Could you check a few things on this model? Use its own coordinates, in mm. Face numbers are marked on the shaded views. A direction names the side the tool comes from. Coordinates: 2 decimals unless noted, no trailing zeros. Loops run counter-clockwise (first coordinate to the right, second up) from the corner with the lowest first, then second, coordinate; pieces in that order, holes last. Notation, with made-up numbers: M 3.25,0.25 L 12.25,0.25 A21 cw 12.25,36.25 Z; hole C 82.25,47.5 d10. An arc over 180 degrees is marked long. Return JSON: item names as keys, results as strings. Group by question number.
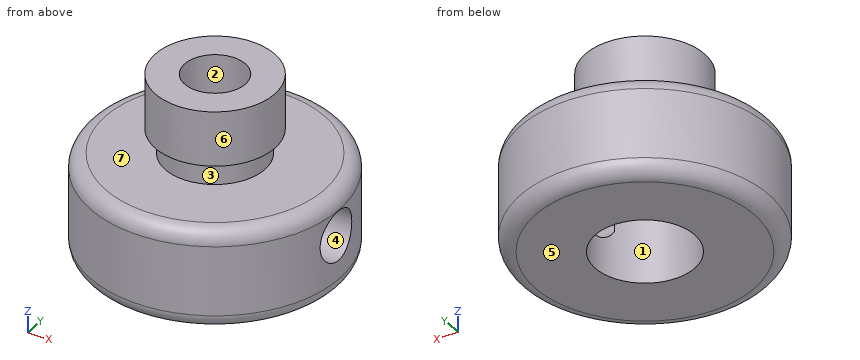
from build123d import *

# Parameters (mm, degrees)
ESQUISSE1_R             = 12.5
BASE_EXTRUSION_DEPTH    = 10
ESQUISSE2_R             = 6
BOSS_EXTRU_1_DEPTH      = 8
ESQUISSE3_R             = 3.05
ENL_V_MAT_EXTRU_1_DEPTH = 26.228951623
ESQUISSE4_R             = 5
ENL_V_MAT_EXTRU_2_DEPTH = 8
ESQUISSE5_W             = 2.5
ESQUISSE5_H             = 2
CONG_1_R                = 1.5
ESQUISSE7_R             = 2.5
ENL_V_MAT_EXTRU_4_DEPTH = 8


with BuildPart() as part:
    # Esquisse1 → Base-Extrusion (new body)
    with BuildSketch(Plane.XY):
        Circle(ESQUISSE1_R)
    extrude(amount=BASE_EXTRUSION_DEPTH)

    # Esquisse2 → Boss.-Extru.1 (add)
    with BuildSketch(Plane.XY.offset(10)):
        Circle(ESQUISSE2_R)
    extrude(amount=BOSS_EXTRU_1_DEPTH)

    # Esquisse3 → Enlèv. mat.-Extru.1 (cut, through all)
    with BuildSketch(Plane.XY.offset(18)):
        Circle(ESQUISSE3_R)
    extrude(amount=-ENL_V_MAT_EXTRU_1_DEPTH, mode=Mode.SUBTRACT)

    # Esquisse4 → Enlèv. mat.-Extru.2 (cut)
    with BuildSketch(Plane(origin=(0, 0, 0), x_dir=(-1, 0, 0), z_dir=(0, 0, -1))):
        Circle(ESQUISSE4_R)
    extrude(amount=-ENL_V_MAT_EXTRU_2_DEPTH, mode=Mode.SUBTRACT)

    # Esquisse5 → Enlever de la matière-Révolution1 (revolve, cut)
    with BuildSketch(Plane(origin=(0, 0, 0), x_dir=(0, 0, -1), z_dir=(1, 0, 0)), mode=Mode.PRIVATE) as enlever_de_la_mati_re_r_volution1_sk:
        with Locations((-11.25, 6)):
            Rectangle(ESQUISSE5_W, ESQUISSE5_H)
    revolve(enlever_de_la_mati_re_r_volution1_sk.sketch.rotate(Axis((0, 0, 21.399826727), (0, 0, -1)), 90), axis=Axis((0, 0, 21.399826727), (0, 0, -1)), mode=Mode.SUBTRACT)

    # Congé1
    cong_1_edges = [part.edges().sort_by_distance(p)[0] for p in [
        (-12.5, 0, 0),
        (-12.5, 0, 10),
    ]]
    fillet(cong_1_edges, radius=CONG_1_R)

    # Esquisse7 → Enlèv. mat.-Extru.4 (cut)
    with BuildSketch(Plane(origin=(12.5, 0, 0), x_dir=(0, 0, -1), z_dir=(1, 0, 0))):
        with Locations((-5.942386831, 0)):
            Circle(ESQUISSE7_R)
    extrude(amount=-ENL_V_MAT_EXTRU_4_DEPTH, mode=Mode.SUBTRACT)


solid = part.part
(1) For the marked faces 5, 6 and 7, which set-ups out of +Z, -Z, +X, -X, +Y, -Y let a thin tool reach every point of the face, with its end or its side?
(2) Imagine slicing it at A-A, the plane x = 0. Write out the boundary of the cut face in (y, z), then the cut area to 3 significant figures.
(3) Will these pins go through, and if not, where does the flat tip stop? P1, Ø1.5, axis at x = 3.5, z = 15, coming from the +Y side; P2, Ø2, axis at x = 3.5, z = 15, coming from the -Y side; P3, Ø1, axis at y = 2.5, z = 5, coming from the -X side; P4, Ø3.5, axis at x = 0, y = 0, coming from the -Z side.
(4) Imagine slicing it at B-B, the plane y = 0. Write out the boundary of the cut face in (x, z).
(5) Imagine slicing it at D-D, the plane z = 11.25. Write out the boundary of the cut face in (x, y).
(6) Imagine slicing it at C-C, the plane z = 14. Write out the boundary of the cut face in (x, y).
(7) We'd pull the mould along X, two halves only. Please class the marked faces 1, 2, 3 and 4: +X half, -X half, draft (parallel to the pull), parting line (faces both ways), or undercut.
(8) If I drill on L1, parallel to Z at x = -5, y = -0.75; L2, parallel to Z at x = 8, y = 0; L3, parallel to Y at x = 0, z = 12.25, over which ranges is the centre line in solid material (lowest first)? Write a range as [from, to].
Checks:
{
 "1": {"face 5": "-Z, +X, -X, +Y, -Y", "face 6": "+Z", "face 7": "none"},
 "2": {"outline": "M -12.5,1.5 A1.5 ccw -11,0 L -5,0 L -5,8 L -3.05,8 L -3.05,18 L -6,18 L -6,12.5 L -5,12.5 L -5,10 L -11,10 A1.5 ccw -12.5,8.5 Z; M 3.05,8 L 5,8 L 5,0 L 11,0 A1.5 ccw 12.5,1.5 L 12.5,8.5 A1.5 ccw 11,10 L 5,10 L 5,12.5 L 6,12.5 L 6,18 L 3.05,18 Z", "area": "198 mm²"},
 "3": {"P1": "y = 5.33", "P2": "y = -5.45", "P3": "x = -12.34", "P4": "through"},
 "4": {"outline": "M -12.5,1.5 A1.5 ccw -11,0 L -5,0 L -5,8 L -3.05,8 L -3.05,18 L -6,18 L -6,12.5 L -5,12.5 L -5,10 L -11,10 A1.5 ccw -12.5,8.5 Z; M 3.05,8 L 4.5,8 L 4.5,8.44 L 12.5,8.44 L 12.5,8.5 A1.5 ccw 11,10 L 5,10 L 5,12.5 L 6,12.5 L 6,18 L 3.05,18 Z; M 5,0 L 11,0 A1.5 ccw 12.5,1.5 L 12.5,3.44 L 5,3.44 Z"},
 "5": {"outline": "C 0,0 d10; hole C 0,0 d6.1"},
 "6": {"outline": "C 0,0 d12; hole C 0,0 d6.1"},
 "7": {"face 1": "undercut", "face 2": "undercut", "face 3": "parting line", "face 4": "draft"},
 "8": {"L1": "[0, 10], [12.5, 18]", "L2": "[0, 3.44], [8.44, 10]", "L3": "[-5, -3.05], [3.05, 5]"}
}
